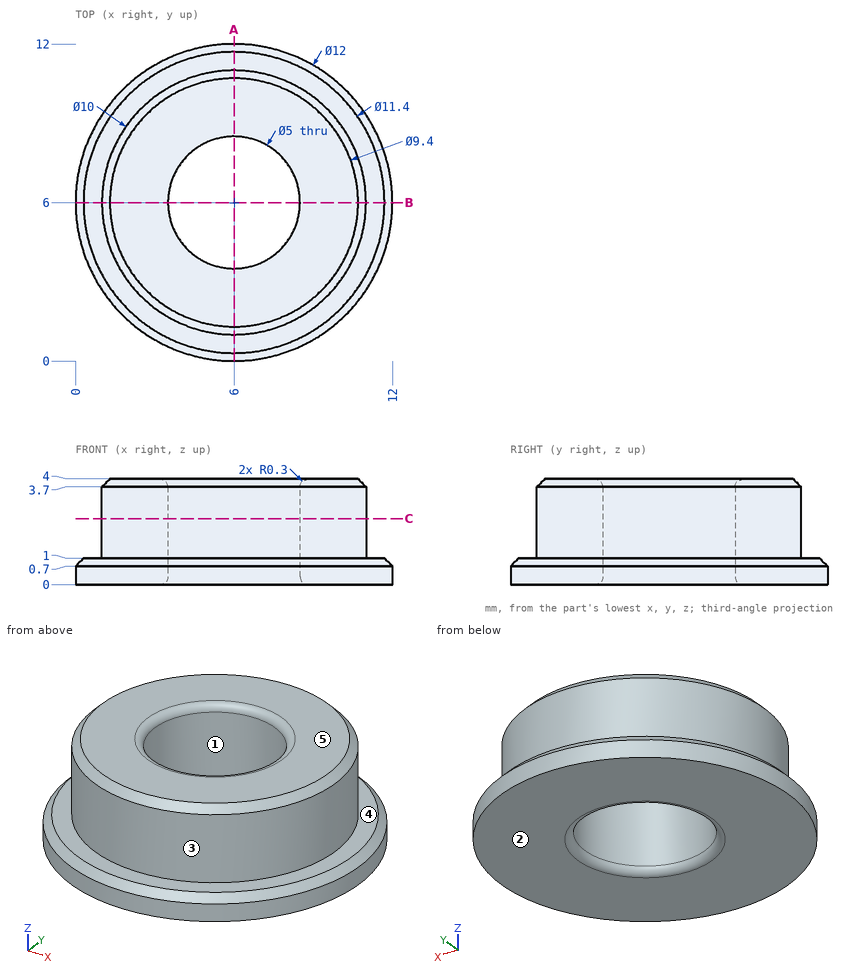
Print and shaded views of the part. All mm, measured from the part's lowest x, y and z. A direction names the side the tool comes from. Round coordinates to 2 decimals unless told otherwise and drop trailing zeros. Write each loop counter-clockwise with the first axis right and the second up, starting at its lowest first coordinate (ties: lowest second). Pieces come first, ordered by that corner, then holes.
(1) Slice it at A-A, the plane x = 6. Write the cut outline in (y, z), and give its area (3 significant figures).
(2) Probe line 1 along Y through (x, z) = (6, 1.05); line 2 along X through (y, z) = (3.75, 0.95); line 3 along Y through (x, z) = (4.75, 1.55). List the from-to ranges inside material, lowest first.
(3) Slice it at C-C, the plane z = 2.5. Write the cut outline in (x, y), and give its area (3 significant figures).
(4) Mould opens along Y. For the marked faces 1, 2 and 3 say: pulls with the +Y half, pulls with the -Y half, needs draft (parallel to the pull), parting line crosses it, or undercut.
(5) Drop flat-ended pins along their axis: P1, Ø4, axis at x = 5.5, y = 4, coming from the +Z side; P2, Ø2, axis at x = 10, z = 0.5, coming from the -Y side. Give the stop position or say it passes through.
(6) 3-axis set-ups, long thin cutter, end or side, ignore diameter. For the marked faces 4 and 5: which of +Z, -Z, +X, -X, +Y, -Y reach the whole face in a straight line?
From the geometry:
1. outline: (0, 0) - (3.2, 0) arc R0.3 ccw to (3.5, 0.3) - (3.5, 3.7) arc R0.3 ccw to (3.2, 4) - (1.3, 4) - (1, 3.7) - (1, 1) - (0.3, 1) - (0, 0.7) - close; (8.5, 0.3) arc R0.3 ccw to (8.8, 0) - (12, 0) - (12, 0.7) - (11.7, 1) - (11, 1) - (11, 3.7) - (10.7, 4) - (8.8, 4) arc R0.3 ccw to (8.5, 3.7) - close
1. area: 21.7 mm2
2. line 1: y = 1 to 3.5, 8.5 to 11
2. line 2: x = 0.71 to 4.91, 7.09 to 11.29
2. line 3: y = 1.16 to 3.83, 8.17 to 10.84
3. outline: circle Ø10 at (6, 6); hole circle Ø5 at (6, 6)
3. area: 58.9 mm2
4. face 1: undercut
4. face 2: needs draft
4. face 3: parting line crosses it
5. P1: stops at z = 4
5. P2: stops at y = 0.8
6. face 4: +Z
6. face 5: +Z, +X, -X, +Y, -Y
